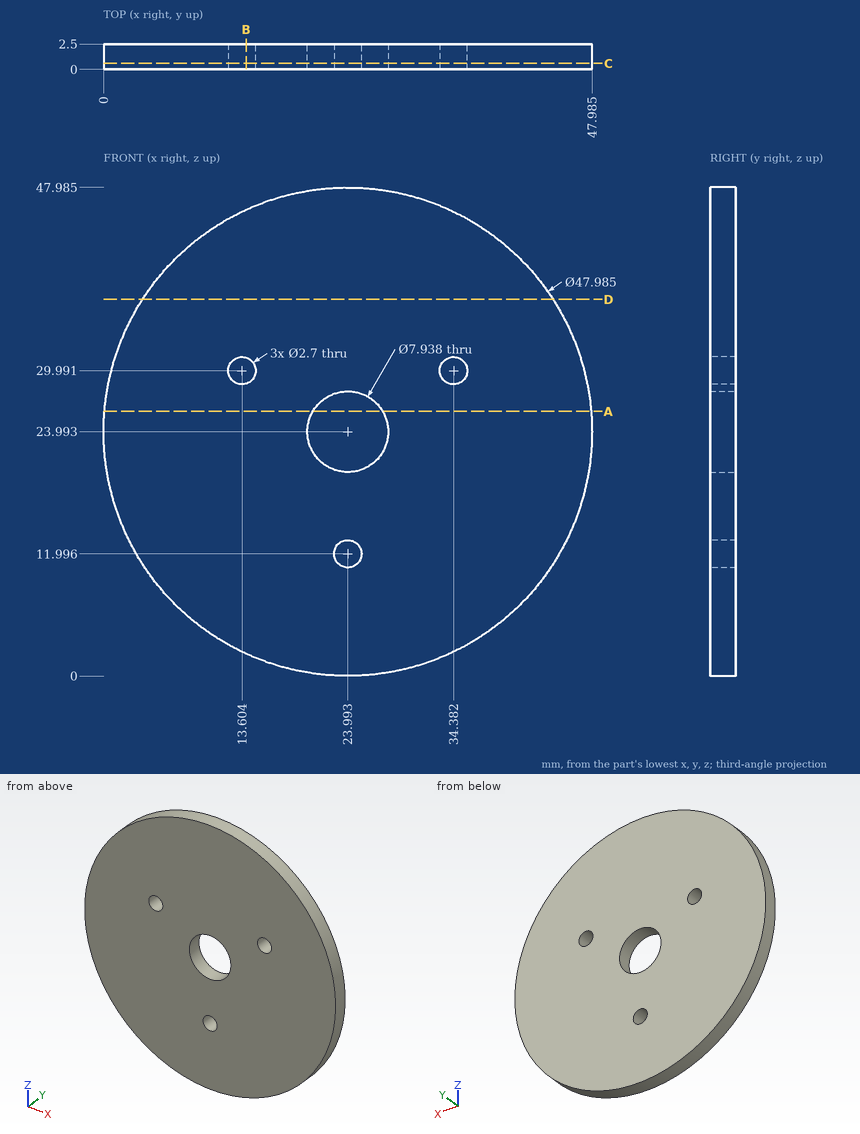
Check sheet for the drawn part. Datum: minimum x, y, z corner. Units: mm. Give positions to 0.01 mm unless a question says otherwise; leave off trailing zeros. Write each loop counter-clockwise with the first axis right and the second up, starting at its lowest first coordinate (ties: lowest second). Pieces come first, ordered by that corner, then holes. Notation, with made-up numbers: M 71.5,63 L 78.5,63 A29 ccw 78.5,96 Z; hole C 61,16.5 d2. An arc over 180 degrees is marked long. Write item = value, one per line.
(1) Material ranges on line 1 (Z direction, x = 24.5, y = 1.05) (1 decimal); line 2 (X direction, y = 0.1, z = 30) (1 decimal); line 3 (X direction, y = 0.1, z = 24) (1 decimal), recorded low to high.
Found:
line_1 = 0 to 10.7, 13.2 to 20.1, 27.9 to 48
line_2 = 0.8 to 12.3, 15 to 33, 35.7 to 47.2
line_3 = 0 to 20, 28 to 48
(2) Sectioned sample at A-A (z = 26). Record the cut outline in (x, y) (1 decimal).
Found:
outline = M 0.1,0 L 20.6,0 L 20.6,2.5 L 0.1,2.5 Z; M 27.4,0 L 47.9,0 L 47.9,2.5 L 27.4,2.5 Z
(3) Sectioned sample at D-D (z = 37). Record the cut outline in (x, y), then the cut area to 3 significant figures.
Found:
outline = M 3.83,0 L 44.15,0 L 44.15,2.5 L 3.83,2.5 Z
area = 101 mm2
(4) Sectioned sample at C-C (y = 0.6). Give the number of separate pieces and of enclosed holes in the cut face, then the cut area to 3 significant figures.
Found:
separate_pieces = 1
enclosed_holes = 4
area = 1,740 mm2
(5) Sectioned sample at B-B (x = 14). Record the cut outline in (y, z) (1 decimal), then the cut area to 3 significant figures.
Found:
outline = M 0,2.2 L 2.5,2.2 L 2.5,28.7 L 0,28.7 Z; M 0,31.3 L 2.5,31.3 L 2.5,45.8 L 0,45.8 Z
area = 103 mm2
